from build123d import *

# Parameters (mm, degrees)
SKETCH_1_R          = 3
EXTRUDE_1_DEPTH     = 37
SKETCH_2_R          = 2.5
CUT_EXTRUDE_1_DEPTH = 6
CHAMFER_1_SIZE      = 1
M3_5X0_61_D         = 2.9


with BuildPart() as part:
    # Эскиз1 → Бобышка-Вытянуть1 (new body)
    with BuildSketch(Plane.XY):
        Circle(SKETCH_1_R)
    extrude(amount=EXTRUDE_1_DEPTH)

    # Эскиз2 → Вырез-Вытянуть1 (cut)
    with BuildSketch(Plane.XY.offset(37)):
        Circle(SKETCH_2_R)
    extrude(amount=-CUT_EXTRUDE_1_DEPTH, mode=Mode.SUBTRACT)

    # Фаска1
    chamfer_1_edges = [part.edges().sort_by_distance(p)[0] for p in [
        (-3, 0, 0),
    ]]
    chamfer(chamfer_1_edges, length=CHAMFER_1_SIZE)

    # Отверстие обработанное метчиком M3.5x0.61 (through all)
    with Locations(Plane(origin=(3, 0, 0), x_dir=(0, 0, -1), z_dir=(1, 0, 0))):
        with Locations((-27, 0)):
            Hole(M3_5X0_61_D / 2)


solid = part.part
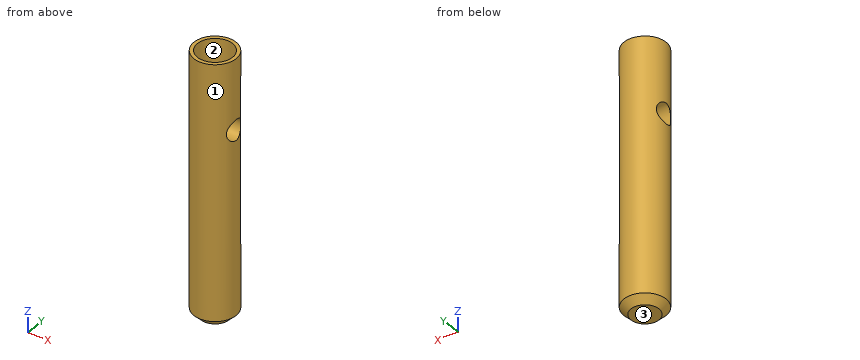
Verification items for the finished model (mm, model axes). Face numbers are marked on the shaded views. Give positions to 0.01 mm unless a question says otherwise; leave off trailing zeros. Loops run counter-clockwise (first coordinate to the right, second up) from the corner with the lowest first, then second, coordinate; pieces in that order, holes last.
1) Sectioned sample at C-C, the plane z = 8.5. Enter the section's corners in (x, y), then the cut area to 3 significant figures.
2) Sectioned sample at B-B, the plane x = 0. Enter the section's corners in (y, z).
3) Sectioned sample at A-A, the plane y = 0. Enter the section's corners in (x, z).
4) Draft check along X on the marked faces 1, 2 and 3. Enter one of: pulls with the +X half, pulls with the -X half, needs draft (parallel to the pull), parting line crosses it, or undercut.
5) Thickness scan on line 1 along Z through (x, y) = (1.5, 0); line 2 along Y through (x, z) = (0.5, 27); line 3 along Y through (x, z) = (0, 34.3). Record the ranges inside material, lowest first.
6) Sectioned sample at D-D, the plane z = 27. Enter the section's corners in (x, y), then the cut area to 3 significant figures.
7) Depth check by flat-ended pin: pin 1 Ø2 at (y, z) = (-1.5, 13.5) entering from -X; pin 2 Ø1 at (x, z) = (1, 8) entering from -Y; pin 3 Ø1.5 at (x, y) = (1, 1) entering from +Z. Enter the tip coordinate at first touch or a pass-through.
Answers:
1. outline: circle Ø6 at (0, 0)
1. area: 28.3 mm2
2. outline: (-3, 1) - (-2, 0) - (2, 0) - (3, 1) - (3, 37) - (2.5, 37) - (2.5, 31) - (-2.5, 31) - (-2.5, 37) - (-3, 37) - close; hole circle Ø2.9 at (0, 27)
3. outline: (-3, 1) - (-2, 0) - (2, 0) - (3, 1) - (3, 25.55) - (-3, 25.55) - close; (-3, 28.45) - (3, 28.45) - (3, 37) - (2.5, 37) - (2.5, 31) - (-2.5, 31) - (-2.5, 37) - (-3, 37) - close
4. face 1: parting line crosses it
4. face 2: undercut
4. face 3: needs draft
5. line 1: z = 0 to 25.55, 28.45 to 31
5. line 2: y = -2.96 to -1.45, 1.45 to 2.96
5. line 3: y = -3 to -2.5, 2.5 to 3
6. outline: (-2.63, -1.45) arc R3 ccw to (2.63, -1.45) - close; (-2.63, 1.45) - (2.63, 1.45) arc R3 ccw to start
6. area: 11.6 mm2
7. pin 1: stops at x = -2.96
7. pin 2: stops at y = -2.96
7. pin 3: stops at z = 31
